from build123d import *

# Parameters (mm, degrees)
BOSS_EXTRUDE1_DEPTH = 16
CUT_EXTRUDE1_DEPTH  = 27.570660511
SKETCH3_R           = 1.6
CUT_EXTRUDE2_DEPTH  = 33.870624557
SKETCH4_R           = 3
CUT_EXTRUDE3_DEPTH  = 27.570660628


with BuildPart() as part:
    # Sketch1 → Boss-Extrude1 (new body)
    with BuildSketch(Plane.XY):
        with BuildLine():
            Line((12.68857754, 8), (13.18857754, 8))
            Line((13.18857754, 8), (13.18857754, -8))
            Line((13.18857754, -8), (12.68857754, -8))
            ThreePointArc((12.68857754, -8), (-15, 0), (12.68857754, 8))
        make_face()
    extrude(amount=BOSS_EXTRUDE1_DEPTH)

    # Sketch2 → Cut-Extrude1 (cut, through all)
    with BuildSketch(Plane.XY.offset(16)):
        with BuildLine():
            Line((-1.638653084, -14.910225219), (-1.638653084, -32.417274257))
            Line((-1.638653084, -32.417274257), (-50.765498106, -32.417274257))
            Line((-50.765498106, -32.417274257), (-50.765498106, 31.239484016))
            Line((-50.765498106, 31.239484016), (12.68857754, 31.239484016))
            Line((12.68857754, 31.239484016), (12.68857754, 8))
            ThreePointArc((12.68857754, 8), (5.024479817, 7.624084306), (-2.566041885, 6.499946049))
            ThreePointArc((-2.566041885, 6.499946049), (-11.285505358, -4.60291117), (-1.638653084, -14.910225219))
        make_face()
    extrude(amount=-CUT_EXTRUDE1_DEPTH, mode=Mode.SUBTRACT)

    # Sketch3 → Cut-Extrude2 (cut, through all)
    with BuildSketch(Plane(origin=(13.18857754, 0, 0), x_dir=(0, 0, -1), z_dir=(1, 0, 0))):
        with Locations((-8, 3.9)):
            Circle(SKETCH3_R)
        with Locations((-8, -3.9)):
            Circle(SKETCH3_R)
    extrude(amount=-CUT_EXTRUDE2_DEPTH, mode=Mode.SUBTRACT)

    # Sketch4 → Cut-Extrude3 (cut, through all)
    with BuildSketch(Plane(origin=(-1.81142246, 0, 0), x_dir=(0, 0, -1), z_dir=(1, 0, 0))):
        with Locations((-8, 3.9)):
            Circle(SKETCH4_R)
        with Locations((-8, -3.9)):
            Circle(SKETCH4_R)
    extrude(amount=-CUT_EXTRUDE3_DEPTH, mode=Mode.SUBTRACT)


solid = part.part
Build history of the part. All positions in model axes, mm. A direction names the side the tool comes from. Coordinates: 2 decimals unless noted, no trailing zeros. Order: outer loops, then holes, each group sorted by start corner. A loop starts at its lowest first (then second) coordinate and runs counter-clockwise, first axis right, second up. Notation, with made-up numbers: (7, 10.25) -> (55, 10.25) arc R21 ccw to (55, 15.25) -> close; hole circle Ø10 at (32, -11.5). An arc over 180 degrees is marked (long way). One line per item, written item: value.
(1) Slice it at B-B, the plane z = 12.5. List the corners of the cut face in (x, y).
Checked values:
outline: (-2.57, 6.5) arc R10.84 ccw to (-1.64, -14.91) arc R15 ccw to (12.69, -8) -> (13.19, -8) -> (13.19, 8) -> (12.69, 8) arc R78.32 ccw to start
(2) Probe line 1 (Z direction, x = 10.75, y = -3.75); line 2 (Y direction, x = -3, z = 10.75); line 3 (Y direction, x = 8.75, z = 8). List the from-to ranges inside material, lowest first. Write a range as [from, to].
Checked values:
line 1: [0, 6.41], [9.59, 16]
line 2: [-14.67, -5.1], [-2.7, 2.7], [5.1, 6.4]
line 3: [-12.18, -5.5], [-2.3, 2.3], [5.5, 7.9]
(3) Slice it at C-C, the plane x = 8. List the corners of the cut face in (y, z), plus the area to 3 significant figures.
Checked values:
outline: (-12.69, 0) -> (7.86, 0) -> (7.86, 16) -> (-12.69, 16) -> close; hole circle Ø3.2 at (-3.9, 8); hole circle Ø3.2 at (3.9, 8)
area: 313 mm2
(4) Slice it at A-A, the plane y = 3.25. List the corners of the cut face in (x, z).
Checked values:
outline: (-8.39, 0) -> (13.19, 0) -> (13.19, 6.54) -> (-1.81, 6.54) -> (-1.81, 5.07) -> (-8.39, 5.07) -> close; (-8.39, 10.93) -> (-1.81, 10.93) -> (-1.81, 9.46) -> (13.19, 9.46) -> (13.19, 16) -> (-8.39, 16) -> close
(5) Slice it at D-D, the plane z = 8. List the corners of the cut face in (x, y), plus the area to 3 significant figures.
Checked values:
outline: (-10.94, -6.9) arc R10.84 ccw to (-1.64, -14.91) arc R15 ccw to (12.69, -8) -> (13.19, -8) -> (13.19, -5.5) -> (-1.81, -5.5) -> (-1.81, -6.9) -> close; (-10.8, -0.9) -> (-1.81, -0.9) -> (-1.81, -2.3) -> (13.19, -2.3) -> (13.19, 2.3) -> (-1.81, 2.3) -> (-1.81, 0.9) -> (-10.06, 0.9) arc R10.84 ccw to start; (-1.81, 5.5) -> (13.19, 5.5) -> (13.19, 8) -> (12.69, 8) arc R78.32 ccw to (-1.81, 6.65) -> close
area: 280 mm2
(6) Mould opens along Z. For faces 1 (the cylindrical face through (6.62, -13.46, 7.89)), 2 (the cylindrical face through (-6.49, -5.05, 5.23)), 3 (the flat face through (1, -3, 0)) say: pulls with the +Z half, pulls with the -Z half, needs draft (parallel to the pull), parting line crosses it, or undercut.
Checked values:
face 1: needs draft
face 2: undercut
face 3: pulls with the -Z half
(7) Tool access for faces 4 (the cylindrical face through (5.79, 3.97, 9.6)), 5 (the cylindrical face through (-5, 0.9, 8.1)): list every direction of +Z, -Z, +X, -X, +Y, -Y with a clear straight run to the whole face (end or side of a thin tool).
Checked values:
face 4: +X, -X
face 5: -X
(8) Drop flat-ended pins along their axis: pin 1 Ø7 at (y, z) = (-3.9, 8) entering from -X; pin 2 Ø4.5 at (y, z) = (4, 9.5) entering from -X; pin 3 Ø5.5 at (y, z) = (3.9, 8) entering from -X; pin 4 Ø5 at (y, z) = (-1.5, 7) entering from -X. Give the stop position or say it passes through.
Checked values:
pin 1: x = -11.3
pin 2: x = -9.49
pin 3: x = -1.81
pin 4: x = -11.25
